Design review of the part built by this model. Coordinates are the model's own, in mm. Face numbers are marked on the shaded views. A direction names the side the tool comes from. Coordinates: 2 decimals unless noted, no trailing zeros. Write each loop counter-clockwise with the first axis right and the second up, starting at its lowest first coordinate (ties: lowest second). Pieces come first, ordered by that corner, then holes. Notation, with made-up numbers: (61.5, -2) - (101.5, -2) arc R24 cw to (101.5, 27) - close; hole circle Ø8 at (19, -24.75). An arc over 180 degrees is marked (long way). Answer as CSV lines item,"result". Start each with the question number.
Q1. We need section B-B (y = 17). Write out the cut boundary in (x, z), plus the area to 3 significant figures.
Q2. Machinability: for the marked faces 4 and 5, which of the approach directions +Z, -Z, +X, -X, +Y, -Y give a long, thin tool a straight path to every point of the face, cutting with its end or side? Answer none if there is none.
Q3. We need section A-A (z = 32). Write out the cut boundary in (x, y) (1 decimal), plus the area to 3 significant figures.
Q4. For line 1 along X through (y, z) = (6, 29); line 2 along Y through (x, z) = (-38, 49) (1 decimal); line 3 along Z through (x, y) = (23, 15.5), list the stretches that pass through material, from the lowest coordinate up. Write a range as [from, to].
Q5. Clearance check with a flat-ended pin moving along its axis: pin 1 (12 mm diameter, centred on x = -30.5, y = 9, fed in from +Z). State where the tip first meets the part, or that it passes through.
Q6. Mouldability with a two-part tool opening along X and no side actions: class the marked faces 1, 2 and 3 as pulls with the +X half, pulls with the -X half, needs draft (parallel to the pull), parting line crosses it, or undercut.
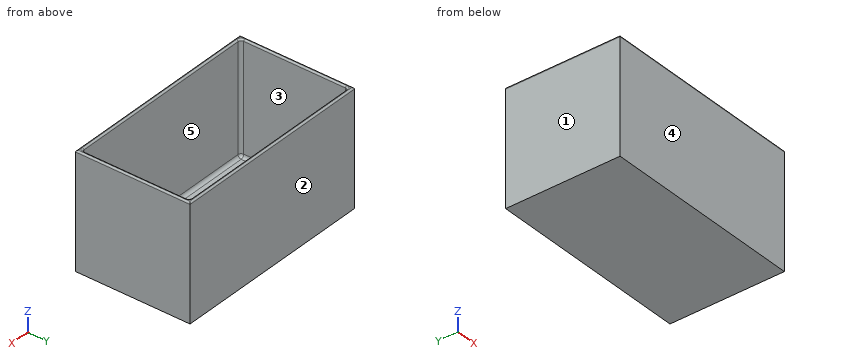
from build123d import *

# Parameters (mm, degrees)
F0_W     = 101.6
F0_H     = 57.15
F0_W_2   = 98.425
F0_H_2   = 53.975
F1_DEPTH = 57.15
F2_DEPTH = 1.5875
F3_R     = 1.5748
F4_R     = 0.762
F5_R     = 20.6375
F6_DEPTH = 6.35


with BuildPart() as f1:
    # F0 (on Top) → F1 (new body)
    with BuildSketch(Plane.XY):
        Rectangle(F0_W, F0_H)
        Rectangle(F0_W_2, F0_H_2, mode=Mode.SUBTRACT)
    extrude(amount=F1_DEPTH)

    # F0 (on Top) → F2 (join)
    with BuildSketch(Plane.XY):
        Rectangle(F0_W_2, F0_H_2)
    extrude(amount=F2_DEPTH)

    # F3
    f3_edges = [f1.edges().sort_by_distance(p)[0] for p in [
        (-49.2125, 26.9875, 29.36875),
        (49.2125, 26.9875, 29.36875),
        (49.2125, -26.9875, 29.36875),
        (49.2125, 0, 1.5875),
        (0, -26.9875, 1.5875),
        (-49.2125, 0, 1.5875),
        (0, 26.9875, 1.5875),
        (-49.2125, -26.9875, 29.36875),
    ]]
    fillet(f3_edges, radius=F3_R)

    # F4
    f4_edges = [f1.edges().sort_by_distance(p)[0] for p in [
        (0, -28.575, 57.15),
        (50.8, 0, 57.15),
        (0, 28.575, 57.15),
        (-50.8, 0, 57.15),
        (-49.2125, 0, 57.15),
    ]]
    fillet(f4_edges, radius=F4_R)


with BuildPart() as f6:
    # F5 (on Front) → F6 (new body)
    with BuildSketch(Plane.XZ):
        with Locations((-50.13819, -40.545423)):
            Circle(F5_R)
    extrude(amount=F6_DEPTH)


solid = f1.part
Results list:
1,outline,"(-50.8, 0) - (50.8, 0) - (50.8, 56.39) arc R0.76 ccw to (50.04, 57.15) - (49.97, 57.15) arc R0.76 ccw to (49.21, 56.39) - (49.21, 3.16) arc R1.57 cw to (47.64, 1.59) - (-47.64, 1.59) arc R1.57 cw to (-49.21, 3.16) - (-49.21, 56.39) arc R0.76 ccw to (-49.97, 57.15) - (-50.04, 57.15) arc R0.76 ccw to (-50.8, 56.39) - close"
1,area,"338 mm2"
2,face 4,"+Z, -Z, +X, -X, -Y"
2,face 5,"+Z"
3,outline,"(-50.8, -28.6) - (50.8, -28.6) - (50.8, 28.6) - (-50.8, 28.6) - close; hole (-49.2, -25.4) arc R1.6 ccw to (-47.6, -27) - (47.6, -27) arc R1.6 ccw to (49.2, -25.4) - (49.2, 25.4) arc R1.6 ccw to (47.6, 27) - (-47.6, 27) arc R1.6 ccw to (-49.2, 25.4) - close"
3,area,"496 mm2"
4,line 1,"x = [-50.8, -49.21], [49.21, 50.8]"
4,line 2,"y = [-28.6, -27], [27, 28.6]"
4,line 3,"z = [0, 1.59]"
5,pin 1,"stops at z = 1.59"
6,face 1,"pulls with the -X half"
6,face 2,"needs draft"
6,face 3,"undercut"
